Part model, mm, in its own coordinate system. A direction names the side the tool comes from. Round coordinates to 2 decimals unless told otherwise and drop trailing zeros. Order: outer loops, then holes, each group sorted by start corner. A loop starts at its lowest first (then second) coordinate and runs counter-clockwise, first axis right, second up. Notation, with made-up numbers: (73, 63.5) -> (80, 63.5) arc R29 cw to (80, 90.5) -> close; hole circle Ø8 at (62.25, 28). An arc over 180 degrees is marked (long way). Use CSV: the item, a comma, the result in double quotes.
Autodesk Fusion 360 part; units mm, degrees
sketch "Sketch1" plane through (0, 0, 0) normal (0, 0, 1) x (1, 0, 0)
  line L0 (21.65, 30) -> (-21.65, 30)
  line L1 (-21.65, 30) -> (-21.65, -30)
  line L2 (-21.65, -30) -> (21.65, -30)
  line L3 (21.65, -30) -> (21.65, 30) construction
  line L4 (21.65, 30) -> (-21.65, -30) construction
  line L5 (-21.65, 30) -> (21.65, -30) construction
  line L6 (0, 30) -> (0, -30) construction
  line L7 (21.65, 0) -> (-21.65, 0) construction
  circle A0 centre (-11.65, 20) radius 1.5
  circle A1 centre (11.65, 20) radius 1.5
  circle A2 centre (-11.65, -20) radius 1.5
  circle A3 centre (11.65, -20) radius 1.5
  line L8 (-6.5, 50.5) -> (35.5, 50.5)
  line L9 (35.5, 50.5) -> (35.5, -50.5)
  line L10 (35.5, -50.5) -> (-6.5, -50.5)
  line L11 (-6.5, -50.5) -> (-6.5, 50.5)
  line L12 (-6.5, 50.5) -> (35.5, -50.5) construction
  line L13 (35.5, 50.5) -> (-6.5, -50.5) construction
  line L14 (-6.5, 0) -> (35.5, 0) construction
  line L15 (31.5, 47.5) -> (-2.5, 47.5)
  line L16 (-2.5, 47.5) -> (-2.5, -47.5)
  line L17 (-2.5, -47.5) -> (31.5, -47.5)
  line L18 (31.5, -47.5) -> (31.5, 47.5)
  line L19 (31.5, 47.5) -> (-2.5, -47.5) construction
  line L20 (-2.5, 47.5) -> (31.5, -47.5) construction
  line L21 (-2.5, 47.5) -> (-2.5, 50.5)
  line L22 (31.5, 47.5) -> (31.5, 50.5)
  line L23 (14.5, 47.5) -> (14.5, -47.5) construction
  line L24 (-6.5, 16) -> (-10.5, 16)
  line L25 (-10.5, 16) -> (-10.5, 10)
  line L26 (-10.5, 10) -> (-6.5, 10)
  line L27 (-6.5, 10) -> (-6.5, 16)
  line L28 (-10.5, -10) -> (-6.5, -10)
  line L29 (-10.5, -16) -> (-10.5, -10)
  line L30 (-6.5, -16) -> (-10.5, -16)
  line L31 (11.65, 20) -> (-6.5, 20) construction
  line L32 (-6.5, 23.26) -> (-6.5, 16.3949)
  line L33 (-2.5, 17.3602) -> (-2.5, 22.9192)
  line L34 (-2.5, 22.9192) -> (-6.5, 16.3949) construction
  line L35 (-6.5, 23.26) -> (-2.5, 17.3602) construction
  line L36 (26, 32.2049) -> (3, 32.2049)
  line L37 (3, 32.2049) -> (3, 47.2049)
  line L38 (3, 47.2049) -> (26, 47.2049)
  line L39 (26, 47.2049) -> (26, 32.2049)
  line L40 (26, 32.2049) -> (3, 47.2049) construction
  line L41 (3, 32.2049) -> (26, 47.2049) construction
  line L42 (3, -47.2049) -> (26, -47.2049)
  line L43 (26, -32.2049) -> (3, -32.2049)
  line L44 (26, -47.2049) -> (26, -32.2049)
  line L45 (3, -32.2049) -> (3, -47.2049)
  line L46 (26, 7.5) -> (3, 7.5)
  line L47 (3, 7.5) -> (3, -7.5)
  line L48 (3, -7.5) -> (26, -7.5)
  line L49 (26, -7.5) -> (26, 7.5)
  line L50 (26, 7.5) -> (3, -7.5) construction
  line L51 (3, 7.5) -> (26, -7.5) construction
  point P0 (14.5, 0)
  point P1 (14.5, 0)
  point P2 (-4.2897, 20)
  point P3 (-4.2897, -20)
  point P4 (14.5, 0)
  point P5 (14.5, 39.7049)
  point P6 (14.5, 0)
  dimension "d1" = 43.3
  dimension "d2" = 60
  dimension "screwHoleThickness" = 3
  dimension "wSpacingScrew" = 11.65
  dimension "lSpacingScrew" = 20
  dimension "width" = 42
  dimension "lengthWall" = 101
  dimension "d8" = 34
  dimension "length" = 95
  dimension "d24" = 14.5
  dimension "screwwallcancel" = 4
  dimension "d26" = 6
  dimension "d27" = 10
  dimension "d43" = 23
  dimension "d44" = 15
  dimension "d45" = 23
  dimension "d46" = 15
extrude "Extrude9" add sketch "Sketch1" along normal blind 2.5 contours L15 L16 L17 L18 L33 | L0 L1 L2 L11 L24 L25 L26 L28 L29 L30 L32 | L8 L15 L21 L22 makes body 1 at (-17.9333, -3.3333, 0) makes body 2 at (21.7167, 19.9016, 0)
extrude "Extrude10" add sketch "Sketch1" along normal blind 32 contours L0 L2 L11 L16 L27 L32 L33 | L0 L8 L11 L16 L21 | L2 L8 L9 L10 L11 L16 L17 L18 L22 bodies 1 2
sketch "Sketch2" plane through (35.5, 0, 0) normal (1, 0, 0) x (0, 1, 0)
  line L0 (-50.5, 0) -> (50.5, 0)
  line L1 (50.5, 0) -> (50.5, 32)
  line L2 (50.5, 32) -> (-50.5, 32)
  line L3 (-50.5, 32) -> (-50.5, 0)
  line L4 (0, 32) -> (0, 0) construction
  line L5 (50.5, 16) -> (-50.5, 16) construction
  line L6 (45.9932, 8.9649) -> (-45.9932, 8.9649)
  line L7 (-45.9932, 8.9649) -> (-45.9932, 23.0351)
  line L8 (-45.9932, 23.0351) -> (45.9932, 23.0351)
  line L9 (45.9932, 23.0351) -> (45.9932, 8.9649)
  line L10 (45.9932, 8.9649) -> (-45.9932, 23.0351) construction
  line L11 (-45.9932, 8.9649) -> (45.9932, 23.0351) construction
  line L12 (-5.1643, 23.0351) -> (-5.1643, 8.9649)
  line L13 (5.1722, 23.0351) -> (5.1722, 8.9649)
  point P0 (0, 16)
sketch "Sketch3" plane through (0, -50.5, 0) normal (0, -1, 0) x (1, 0, 0)
  line L0 (-6.5, 0) -> (35.5, 0)
  line L1 (35.5, 0) -> (35.5, 32)
  line L2 (35.5, 32) -> (-6.5, 32)
  line L3 (-6.5, 32) -> (-6.5, 0)
  line L4 (14.5, 32) -> (14.5, 0) construction
  line L5 (35.5, 16) -> (-6.5, 16) construction
  line L6 (29.9102, 8.8033) -> (-0.9102, 8.8033)
  line L7 (-0.9102, 8.8033) -> (-0.9102, 23.1967)
  line L8 (-0.9102, 23.1967) -> (29.9102, 23.1967)
  line L9 (29.9102, 23.1967) -> (29.9102, 8.8033)
  line L10 (29.9102, 8.8033) -> (-0.9102, 23.1967) construction
  line L11 (-0.9102, 8.8033) -> (29.9102, 23.1967) construction
  point P0 (14.5, 16)
extrude "Extrude11" cut sketch "Sketch3" against normal blind 3 contours L6 L7 L8 L9 bodies 1
extrude "Extrude12" cut sketch "Sketch2" against normal blind 4 contours L6 L8 L9 L13 | L6 L8 L12 L13 | L6 L7 L8 L12 bodies 1
sketch "Sketch4" plane through (-6.5, 0, 0) normal (-1, 0, 0) x (0, -1, 0)
  line L0 (-10, 0) -> (-10, 2.5)
  line L1 (-10, 2.5) -> (10, 2.5)
  line L2 (10, 2.5) -> (10, 0)
  line L3 (10, 0) -> (16, 0)
  line L4 (16, 0) -> (16, 2.5)
  line L5 (16, 2.5) -> (30, 2.5)
  line L6 (30, 2.5) -> (30, 0)
  line L7 (30, 0) -> (50.5, 0)
  line L8 (50.5, 0) -> (50.5, 32)
  line L9 (50.5, 32) -> (-50.5, 32)
  line L10 (-50.5, 32) -> (-50.5, 0)
  line L11 (-50.5, 0) -> (-30, 0)
  line L12 (-30, 0) -> (-30, 2.5)
  line L13 (-30, 2.5) -> (-16, 2.5)
  line L14 (-16, 2.5) -> (-16, 0)
  line L15 (-16, 0) -> (-10, 0)
  line L16 (0, 32) -> (0, 0) construction
  line L17 (50.5, 16) -> (-50.5, 16) construction
  line L18 (39.9916, 22.0397) -> (-39.9916, 22.0397)
  line L19 (-39.9916, 22.0397) -> (-39.9916, 9.9603)
  line L20 (-39.9916, 9.9603) -> (39.9916, 9.9603)
  line L21 (39.9916, 9.9603) -> (39.9916, 22.0397)
  line L22 (39.9916, 22.0397) -> (-39.9916, 9.9603) construction
  line L23 (-39.9916, 22.0397) -> (39.9916, 9.9603) construction
  line L24 (-7.0931, 22.0397) -> (8.6732, 22.0397)
  line L25 (8.6732, 22.0397) -> (8.6732, 9.9603)
  line L26 (8.6732, 9.9603) -> (-7.0931, 9.9603)
  line L27 (-7.0931, 9.9603) -> (-7.0931, 22.0397)
  point P0 (0, 16)
extrude "Extrude13" cut sketch "Sketch4" against normal blind 4 contours L18 L20 L21 L25 | L18 L20 L24 L25 L26 L27 | L18 L19 L20 L27 bodies 1
sketch "Sketch5" plane through (0, 0, 2.5) normal (0, 0, 1) x (-1, 0, 0)
  line L0 (-3, 47.2049) -> (-3, 32.2049)
  line L1 (-3, 32.2049) -> (-26, 32.2049)
  line L2 (-26, 32.2049) -> (-26, 47.2049)
  line L3 (-26, 47.2049) -> (-3, 47.2049)
  line L4 (-3, -47.2049) -> (-26, -47.2049)
  line L5 (-26, -47.2049) -> (-26, -32.2049)
  line L6 (-26, -32.2049) -> (-3, -32.2049)
  line L7 (-3, -32.2049) -> (-3, -47.2049)
  circle A0 centre (-11.65, -20) radius 1.5
  circle A1 centre (-11.65, 20) radius 1.5
  line L8 (-26, -7.5) -> (-26, 7.5)
  line L9 (-26, 7.5) -> (-3, 7.5)
  line L10 (-3, 7.5) -> (-3, -7.5)
  line L11 (-3, -7.5) -> (-26, -7.5)
  line L12 (2.5, 47.5) -> (-31.5, 47.5)
  line L13 (-31.5, 47.5) -> (-31.5, -50.5)
  line L14 (-31.5, -50.5) -> (2.5, -50.5)
  line L15 (2.5, -50.5) -> (2.5, 47.5)
  circle A2 centre (-11.65, -20) radius 4
  circle A3 centre (-11.65, 20) radius 4
  dimension "d57" = 8
  dimension "d58" = 8
extrude "Extrude14" cut sketch "Sketch5" against normal blind 0.5 contours A2 | A3 bodies 1
sketch "Sketch6" plane through (0, 0, 32) normal (0, 0, 1) x (-1, 0, 0)
  line L0 (2.5, 47.5) -> (2.5, -50.5)
  line L1 (2.5, -50.5) -> (6.5, -50.5)
  line L2 (6.5, -50.5) -> (6.5, 50.5)
  line L3 (6.5, 50.5) -> (-35.5, 50.5)
  line L4 (-35.5, 50.5) -> (-35.5, -50.5)
  line L5 (-35.5, -50.5) -> (-31.5, -50.5)
  line L6 (-31.5, -50.5) -> (-31.5, 47.5)
  line L7 (-31.5, 47.5) -> (2.5, 47.5)
  line L8 (6.5, -50.5) -> (-35.5, -50.5)
  line L9 (-35.5, -50.5) -> (-35.5, 50.5)
  line L10 (-35.5, 50.5) -> (6.5, 50.5)
  line L11 (6.5, 50.5) -> (6.5, -50.5)
  line L12 (2.5, -41.6336) -> (-31.5, -41.6336)
  line L13 (-31.5, -41.6336) -> (-31.5, -11.6336)
  line L14 (-31.5, -11.6336) -> (2.5, -11.6336)
  line L15 (2.5, -11.6336) -> (2.5, -41.6336)
  line L16 (2.5, 11.6067) -> (-31.5, 11.6067)
  line L17 (-31.5, 11.6067) -> (-31.5, 41.6067)
  line L18 (-31.5, 41.6067) -> (2.5, 41.6067)
  line L19 (2.5, 41.6067) -> (2.5, 11.6067)
  line L20 (-8, -49) -> (-21, -49)
  line L21 (-21, -49) -> (-21, -38)
  line L22 (-21, -38) -> (-8, -38)
  line L23 (-8, -38) -> (-8, -49)
  line L24 (-10, 37) -> (-21, 37)
  line L25 (-21, 37) -> (-21, 46)
  line L26 (-21, 46) -> (-10, 46)
  line L27 (-10, 46) -> (-10, 37)
  line L28 (2.5, -0.0134) -> (-31.5, -0.0134) construction
  line L29 (-3, -8) -> (-26, -8)
  line L30 (-26, -8) -> (-26, 8)
  line L31 (-26, 8) -> (-3, 8)
  line L32 (-3, 8) -> (-3, -8)
  dimension "d63" = 30
  dimension "d64" = 30
extrude "Extrude15" add sketch "Sketch6" along normal blind 1 contours L0 L1 L2 L3 L4 L5 L6 L7 L8 L9 L10 L11 L13 L15 L17 L19 | L0 L6 L7 L18 L25 L26 L27 | L0 L6 L14 L16 | L0 L6 L8 L12 L20 L21 L23 | L29 L30 L31 L32 bodies 1
extrude "Extrude16" cut sketch "Sketch6" along normal blind 2 contours L29 L30 L31 L32 bodies 1
extrude "Extrude17" add sketch "Sketch2" against normal blind 3 contours L6 L8 L12 L13 bodies 1
extrude "Extrude18" add sketch "Sketch4" against normal blind 3 contours L18 L20 L24 L25 L26 L27 bodies 1
extrude "Extrusion19" cut 2 faces at (8.5038, 20.2732, 2) (8.5038, -19.7268, 2) along direction (0, 0, -1) blind 0.5 on bodies 1 bodies 1
equation "d1 = 10 mm + 23.3 mm + 10 mm"
equation "d2 = 10 mm + 40 mm + 10 mm"
equation "width = 36 mm + 2 * wallThickness"
equation "lengthWall = length + 2 * wallThickness"
equation "wallThickness = 3 mm"
(1) Drop flat-ended pins along their axis: P1, Ø4, axis at x = 25.5, y = 29.5, coming from the +Z side; P2, Ø8.5, axis at y = 0, z = 12.5, coming from the -X side. Give the stop position or say it passes through.
Reply:
P1,"z = 2.5"
P2,"x = -6.5"
(2) Cut at A-A, the plane y = 15. Give the cut face in (x, z).
Reply:
outline,"(-21.65, 0) -> (-10.5, 0) -> (-10.5, 2.5) -> (-21.65, 2.5) -> close; (-6.5, 0) -> (35.5, 0) -> (35.5, 8.96) -> (31.5, 8.96) -> (31.5, 2.5) -> (-2.5, 2.5) -> (-2.5, 9.96) -> (-6.5, 9.96) -> close; (-6.5, 22.04) -> (-2.5, 22.04) -> (-2.5, 33) -> (-6.5, 33) -> close; (31.5, 23.04) -> (35.5, 23.04) -> (35.5, 33) -> (31.5, 33) -> close"
(3) Cut at D-D, the plane y = -20. State how many separate pieces and enclosed holes the cut face has, then the cut area to 3 significant figures.
Reply:
separate pieces,"5"
enclosed holes,"0"
area,"262 mm2"
(4) Probe probe 1 along X at (y, z) = (19, 5); probe 2 along X at (y, z) = (11, 2); probe 3 along Y at (x, z) = (-11, 1). List the from-to ranges inside material, lowest first. Write a range as [from, to].
Reply:
probe 1,"[-6.5, -2.5], [31.5, 35.5]"
probe 2,"[-21.65, -10.5], [-6.5, 35.5]"
probe 3,"[-30, -21.35], [-18.65, 18.65], [21.35, 30]"
(5) Which spindle directions (+Z, -Z, +X, -X, +Y, -Y) get a long thin tool onto all of the face, cutting with end or side? Do faces 3 (the face through (-5, -8.673, 16)), 4 (the face through (26, 40, 1)), 5 (the face through (32.5, 0, 16)), 6 (the face through (12.171, 16.034, 2.007)). Say none if no direction does.
Reply:
face 3,"+X, -X"
face 4,"-Z"
face 5,"none"
face 6,"+Z"
(6) Pull direction Y, two halves, no side cores. Call faces 1 (the face through (-8, -16, 1)), 2 (the face through (29.91, -49, 16)): released by +Y, released by -Y, zero draft, split by the parting line, or undercut.
Reply:
face 1,"undercut"
face 2,"zero draft"
(7) Cut at C-C, the plane z = 28.5. Give the cut face in (x, y).
Reply:
outline,"(-6.5, -50.5) -> (35.5, -50.5) -> (35.5, 50.5) -> (31.5, 50.5) -> (31.5, -47.5) -> (-2.5, -47.5) -> (-2.5, 50.5) -> (-6.5, 50.5) -> close"
(8) Cut at B-B, the plane x = 27. Give the cut face in (y, z).
Reply:
outline,"(-50.5, 0) -> (50.5, 0) -> (50.5, 2.5) -> (-47.5, 2.5) -> (-47.5, 8.8) -> (-50.5, 8.8) -> close; (-50.5, 23.2) -> (-47.5, 23.2) -> (-47.5, 32) -> (-41.61, 32) -> (-41.61, 33) -> (-50.5, 33) -> close; (-11.61, 32) -> (11.63, 32) -> (11.63, 33) -> (-11.61, 33) -> close; (41.63, 32) -> (50.5, 32) -> (50.5, 33) -> (41.63, 33) -> close"
